from build123d import *

# Parameters (mm, degrees)
F0_W     = 27
F0_H     = 9
F1_DEPTH = 12
F2_R     = 6.25
F3_DEPTH = 9.001
F4_R     = 8.25
F5_DEPTH = 3
F6_R     = 2.1
F7_DEPTH = 12.001


with BuildPart() as f1:
    # F0 (on Front) → F1 (new body)
    with BuildSketch(Plane.XZ):
        with Locations((-1.5, 4.5)):
            Rectangle(F0_W, F0_H)
    extrude(amount=F1_DEPTH)

    # F2 (on face) → F3 (cut, through all)
    with BuildSketch(Plane.XY.offset(9)):
        Circle(F2_R)
    extrude(amount=-F3_DEPTH, mode=Mode.SUBTRACT)

    # F4 (on face) → F5 (cut)
    with BuildSketch(Plane(origin=(0, 0, 0), x_dir=(1, 0, 0), z_dir=(0, 0, -1))):
        Circle(F4_R)
    extrude(amount=-F5_DEPTH, mode=Mode.SUBTRACT)

    # F6 (on face) → F7 (cut, through all)
    with BuildSketch(Plane(origin=(0, 0, 0), x_dir=(-1, 0, 0), z_dir=(0, 1, 0))):
        with Locations((-9.25, 6)):
            Circle(F6_R)
        with Locations((9.25, 6)):
            Circle(F6_R)
    extrude(amount=-F7_DEPTH, mode=Mode.SUBTRACT)


solid = f1.part
The listing builds one solid part. Answer for the finished solid, in the listing's coordinates (mm). A direction names the side the tool comes from. Give positions to 0.01 mm unless a question says otherwise; leave off trailing zeros. Loops run counter-clockwise (first coordinate to the right, second up) from the corner with the lowest first, then second, coordinate; pieces in that order, holes last.
Item 1: A tool of negligible diameter and unlimited length cuts with its end or side. For faces 1 (the flat face through (-2, -7, 9)), 2 (the flat face through (0, -7, 3)), from which of +Z, -Z, +X, -X, +Y, -Y can it reach the whole face along a straight path? Write none if from no direction.
Derived:
face 1: +Z, +X, -X, +Y, -Y
face 2: -Z, +Y
Item 2: A cutting plane is placed at D-D (x = 0). Give the vertices of the cut face in (y, z), then the cut area to 4 significant figures.
Derived:
outline: (-12, 0) - (-8.25, 0) - (-8.25, 3) - (-6.25, 3) - (-6.25, 9) - (-12, 9) - close
area: 45.75 mm2
Item 3: Determine the mould class of faces 3 (the flat face through (12, -6, 4)), 4 (the cylindrical face through (-7.702, -5.916, 7.419)), 5 (the flat face through (-2, -9, 0)) for opening direction X: +X half, -X half, draft (parallel to the pull), parting line (faces both ways), or undercut.
Derived:
face 3: +X half
face 4: undercut
face 5: draft
Item 4: A cutting plane is placed at A-A (x = 9.25). Give the vertices of the cut face in (y, z), then the cut area to 3 significant figures.
Derived:
outline: (-12, 0) - (0, 0) - (0, 3.9) - (-12, 3.9) - close; (-12, 8.1) - (0, 8.1) - (0, 9) - (-12, 9) - close
area: 57.6 mm2
Item 5: Find the intervals of material crossed by line 1 along Z through (x, y) = (9.25, -3.25); line 2 along Z through (x, y) = (-6, -3.5); line 3 along X through (y, z) = (-7.5, 5.5), in increasing order.
Derived:
line 1: z = 0 to 3.9, 8.1 to 9
line 2: z = 3 to 9
line 3: x = -15 to -11.29, -7.21 to 7.21, 11.29 to 12
Item 6: A cutting plane is placed at B-B (y = -1.25). Give the vertices of the cut face in (x, z), then the cut area to 3 significant figures.
Derived:
outline: (-15, 0) - (-8.15, 0) - (-8.15, 3) - (-6.12, 3) - (-6.12, 9) - (-15, 9) - close; (6.12, 3) - (8.15, 3) - (8.15, 0) - (12, 0) - (12, 9) - (6.12, 9) - close; hole circle Ø4.2 at (-9.25, 6); hole circle Ø4.2 at (9.25, 6)
area: 92.9 mm2
Item 7: This flat-tipped pin is pushed along its axis until it touches: pin 1 Ø1 at (x, z) = (0, 1.5) entering from +Y. Where does it stop, or does it pass through?
Derived:
pin 1: stops at y = -8.23
Item 8: A cutting plane is placed at C-C (z = 4.25). Give the vertices of the cut face in (x, y).
Derived:
outline: (-15, -12) - (-10.41, -12) - (-10.41, 0) - (-15, 0) - close; (-8.09, -12) - (8.09, -12) - (8.09, 0) - (6.25, 0) arc R6.25 cw to (-6.25, 0) - (-8.09, 0) - close; (10.41, -12) - (12, -12) - (12, 0) - (10.41, 0) - close
